The listing builds one solid part. Answer for the finished solid, in the listing's coordinates (mm). A direction names the side the tool comes from. Give positions to 0.01 mm unless a question says otherwise; leave off trailing zeros. Loops run counter-clockwise (first coordinate to the right, second up) from the corner with the lowest first, then second, coordinate; pieces in that order, holes last. Notation, with made-up numbers: M 44.5,1.5 L 82.5,1.5 A22 ccw 82.5,38.5 Z; hole C 75,41 d4. An arc over 180 degrees is marked long. Return JSON: item names as keys, results as strings.
from build123d import *

# Parameters (mm, degrees)
SKETCH_1_W          = 270
SKETCH_1_H          = 60
EXTRUDE_1_DEPTH     = 3
SKETCH_2_R          = 2.15
SKETCH_2_R_2        = 1.6
CUT_EXTRUDE_1_DEPTH = 3
SKETCH_3_R          = 1.6
CUT_EXTRUDE_2_DEPTH = 10
CUT_EXTRUDE_3_DEPTH = 10
FILLET_1_R          = 3
FILLET_2_R          = 4
SKETCH_5_W          = 100
SKETCH_5_H          = 40
CUT_EXTRUDE_4_DEPTH = 10
EXTRUDE_2_DEPTH     = 3
EXTRUDE_9_DEPTH     = 3
EXTRUDE_10_DEPTH    = 3
EXTRUDE_11_DEPTH    = 3
EXTRUDE_13_DEPTH    = 3
EXTRUDE_14_DEPTH    = 3
EXTRUDE_16_DEPTH    = 3
EXTRUDE_17_DEPTH    = 3
EXTRUDE_18_DEPTH    = 3
EXTRUDE_19_DEPTH    = 3
CUT_EXTRUDE_5_DEPTH = 4
FILLET_4_R          = 4


with BuildPart() as part:
    # 草图1 → 凸台-拉伸1 (new body)
    with BuildSketch(Plane(origin=(0, 0, 0), x_dir=(1, 0, 0), z_dir=(0, 1, 0))):
        Rectangle(SKETCH_1_W, SKETCH_1_H)
    extrude(amount=EXTRUDE_1_DEPTH)

    # 草图2 → 切除-拉伸1 (cut)
    with BuildSketch(Plane(origin=(0, 3, 0), x_dir=(1, 0, 0), z_dir=(0, 1, 0))):
        with Locations((-23, 0)):
            Circle(SKETCH_2_R)
        with Locations((23, 0)):
            Circle(SKETCH_2_R)
        with Locations((-125, -20)):
            Circle(SKETCH_2_R_2)
        with Locations((-125, -60)):
            Circle(SKETCH_2_R_2)
        with Locations((125, -60)):
            Circle(SKETCH_2_R_2)
        with Locations((125, -20)):
            Circle(SKETCH_2_R_2)
    extrude(amount=-CUT_EXTRUDE_1_DEPTH, mode=Mode.SUBTRACT)

    # 草图3 → 切除-拉伸2 (cut)
    with BuildSketch(Plane(origin=(0, 3, 0), x_dir=(1, 0, 0), z_dir=(0, 1, 0))):
        with Locations((125, 20)):
            Circle(SKETCH_3_R)
        with Locations((100, 20)):
            Circle(SKETCH_3_R)
        with Locations((75, 20)):
            Circle(SKETCH_3_R)
        with Locations((0, 20)):
            Circle(SKETCH_3_R)
        with Locations((-75, 20)):
            Circle(SKETCH_3_R)
        with Locations((-100, 20)):
            Circle(SKETCH_3_R)
        with Locations((-125, 20)):
            Circle(SKETCH_3_R)
    extrude(amount=-CUT_EXTRUDE_2_DEPTH, mode=Mode.SUBTRACT)

    # 草图4 → 切除-拉伸3 (cut)
    with BuildSketch(Plane(origin=(0, 3, 0), x_dir=(1, 0, 0), z_dir=(0, 1, 0))):
        with BuildLine():
            Line((-112.832473586, 10.419213325), (-112.99590583, 10.347711719))
            ThreePointArc((-112.99590583, 10.347711719), (-119.580786675, 12.924404223), (-117.00409417, 19.509285068))
            Line((-117.00409417, 19.509285068), (-116.840661926, 19.580786675))
            ThreePointArc((-116.840661926, 19.580786675), (-110.255781081, 17.00409417), (-112.832473586, 10.419213325))
        make_face()
        with BuildLine():
            Line((-79.771332565, 7.419213325), (-112.99590583, -7.116537478))
            ThreePointArc((-112.99590583, -7.116537478), (-119.580786675, -4.539844974), (-117.00409417, 2.045035871))
            Line((-117.00409417, 2.045035871), (-83.779520905, 16.580786675))
            ThreePointArc((-83.779520905, 16.580786675), (-77.194640061, 14.00409417), (-79.771332565, 7.419213325))
        make_face()
        with BuildLine():
            Line((-32.99590583, 10.419213325), (-112.99590583, -24.580786675))
            ThreePointArc((-112.99590583, -24.580786675), (-119.580786675, -22.00409417), (-117.00409417, -15.419213325))
            Line((-117.00409417, -15.419213325), (-37.00409417, 19.580786675))
            ThreePointArc((-37.00409417, 19.580786675), (-30.419213325, 17.00409417), (-32.99590583, 10.419213325))
        make_face()
        with BuildLine():
            Line((-32.99590583, -10.045035871), (-66.220479095, -24.580786675))
            ThreePointArc((-66.220479095, -24.580786675), (-72.805359939, -22.00409417), (-70.228667435, -15.419213325))
            Line((-70.228667435, -15.419213325), (-37.00409417, -0.883462522))
            ThreePointArc((-37.00409417, -0.883462522), (-30.419213325, -3.460155026), (-32.99590583, -10.045035871))
        make_face()
        with BuildLine():
            Line((-32.99590583, -24.509285068), (-33.159338074, -24.580786675))
            ThreePointArc((-33.159338074, -24.580786675), (-39.744218919, -22.00409417), (-37.167526414, -15.419213325))
            Line((-37.167526414, -15.419213325), (-37.00409417, -15.347711719))
            ThreePointArc((-37.00409417, -15.347711719), (-30.419213325, -17.924404223), (-32.99590583, -24.509285068))
        make_face()
        with BuildLine():
            Line((32.99590583, -24.509285068), (33.159338074, -24.580786675))
            ThreePointArc((33.159338074, -24.580786675), (39.744218919, -22.00409417), (37.167526414, -15.419213325))
            Line((37.167526414, -15.419213325), (37.00409417, -15.347711719))
            ThreePointArc((37.00409417, -15.347711719), (30.419213325, -17.924404223), (32.99590583, -24.509285068))
        make_face()
        with BuildLine():
            Line((32.99590583, -10.045035871), (66.220479095, -24.580786675))
            ThreePointArc((66.220479095, -24.580786675), (72.805359939, -22.00409417), (70.228667435, -15.419213325))
            Line((70.228667435, -15.419213325), (37.00409417, -0.883462522))
            ThreePointArc((37.00409417, -0.883462522), (30.419213325, -3.460155026), (32.99590583, -10.045035871))
        make_face()
        with BuildLine():
            Line((32.99590583, 10.419213325), (112.99590583, -24.580786675))
            ThreePointArc((112.99590583, -24.580786675), (119.580786675, -22.00409417), (117.00409417, -15.419213325))
            Line((117.00409417, -15.419213325), (37.00409417, 19.580786675))
            ThreePointArc((37.00409417, 19.580786675), (30.419213325, 17.00409417), (32.99590583, 10.419213325))
        make_face()
        with BuildLine():
            Line((79.771332565, 7.419213325), (112.99590583, -7.116537478))
            ThreePointArc((112.99590583, -7.116537478), (119.580786675, -4.539844974), (117.00409417, 2.045035871))
            Line((117.00409417, 2.045035871), (83.779520905, 16.580786675))
            ThreePointArc((83.779520905, 16.580786675), (77.194640061, 14.00409417), (79.771332565, 7.419213325))
        make_face()
        with BuildLine():
            Line((112.832473586, 10.419213325), (112.99590583, 10.347711719))
            ThreePointArc((112.99590583, 10.347711719), (119.580786675, 12.924404223), (117.00409417, 19.509285068))
            Line((117.00409417, 19.509285068), (116.840661926, 19.580786675))
            ThreePointArc((116.840661926, 19.580786675), (110.255781081, 17.00409417), (112.832473586, 10.419213325))
        make_face()
        Polygon((0, -20), (-22.5, -20), (0, 0), (22.5, -20), align=None)
    extrude(amount=-CUT_EXTRUDE_3_DEPTH, mode=Mode.SUBTRACT)

    # 圆角1
    fillet_1_edges = [part.edges().sort_by_distance(p)[0] for p in [
        (22.5, 1.5, 20),
        (-22.5, 1.5, 20),
        (0, 1.5, 0),
    ]]
    fillet(fillet_1_edges, radius=FILLET_1_R)

    # 圆角2
    fillet_2_edges = [part.edges().sort_by_distance(p)[0] for p in [
        (135, 1.5, 30),
        (-135, 1.5, 30),
        (-135, 1.5, -30),
        (135, 1.5, -30),
    ]]
    fillet(fillet_2_edges, radius=FILLET_2_R)

    # 草图5 → 切除-拉伸4 (cut)
    with BuildSketch(Plane(origin=(0, 3, 0), x_dir=(1, 0, 0), z_dir=(0, 1, 0))):
        with Locations((-85, -10)):
            Rectangle(SKETCH_5_W, SKETCH_5_H)
        with Locations((85, -10)):
            Rectangle(SKETCH_5_W, SKETCH_5_H)
    extrude(amount=-CUT_EXTRUDE_4_DEPTH, mode=Mode.SUBTRACT)

    # 草图6 → 凸台-拉伸2 (add)
    with BuildSketch(Plane(origin=(0, 3, 0), x_dir=(1, 0, 0), z_dir=(0, 1, 0))):
        with BuildLine():
            Line((-111.519942965, 10), (-118.153192546, 10))
            ThreePointArc((-118.153192546, 10), (-114.836567756, 21), (-111.519942965, 10))
        make_face()
    extrude(amount=-EXTRUDE_2_DEPTH)

    # 草图7 → 凸台-拉伸9 (add)
    with BuildSketch(Plane(origin=(0, 3, 0), x_dir=(1, 0, 0), z_dir=(0, 1, 0))):
        with BuildLine():
            Line((-98.821319018, 10), (-83.779520905, 16.580786675))
            ThreePointArc((-83.779520905, 16.580786675), (-78.241472851, 15.537113222), (-77.19285104, 10))
            Line((-77.19285104, 10), (-98.821319018, 10))
        make_face()
    extrude(amount=-EXTRUDE_9_DEPTH)

    # 草图8 → 凸台-拉伸10 (add)
    with BuildSketch(Plane(origin=(0, 3, 0), x_dir=(1, 0, 0), z_dir=(0, 1, 0))):
        with BuildLine():
            Line((-58.90303514, 10), (-35, 9.542422126))
            Line((-35, 9.542422126), (-32.99590583, 10.419213325))
            ThreePointArc((-32.99590583, 10.419213325), (-30.419213325, 17.00409417), (-37.00409417, 19.580786675))
            Line((-37.00409417, 19.580786675), (-58.90303514, 10))
        make_face()
    extrude(amount=-EXTRUDE_10_DEPTH)

    # 草图9 → 凸台-拉伸11 (add)
    with BuildSketch(Plane(origin=(0, 3, 0), x_dir=(1, 0, 0), z_dir=(0, 1, 0))):
        with BuildLine():
            Line((-35, -0.464249197), (-35, -10.921827071))
            Line((-35, -10.921827071), (-32.99590583, -10.045035871))
            ThreePointArc((-32.99590583, -10.045035871), (-30.105925349, -4.440514214), (-35, -0.464249197))
        make_face()
    extrude(amount=-EXTRUDE_11_DEPTH)

    # 草图10 → 凸台-拉伸13 (add)
    with BuildSketch(Plane(origin=(0, 3, 0), x_dir=(1, 0, 0), z_dir=(0, 1, 0))):
        with BuildLine():
            Line((-35, -14.928498393), (-35, -24.997328276))
            ThreePointArc((-35, -24.997328276), (-29.965585058, -19.962913335), (-35, -14.928498393))
        make_face()
    extrude(amount=-EXTRUDE_13_DEPTH)

    # 草图11 → 凸台-拉伸14 (add)
    with BuildSketch(Plane(origin=(0, 3, 0), x_dir=(1, 0, 0), z_dir=(0, 1, 0))):
        with BuildLine():
            Line((35, -0.464249197), (35, -10.921827071))
            ThreePointArc((35, -10.921827071), (29.771211063, -5.693038134), (35, -0.464249197))
        make_face()
    extrude(amount=-EXTRUDE_14_DEPTH)

    # 草图12 → 凸台-拉伸16 (add)
    with BuildSketch(Plane(origin=(0, 3, 0), x_dir=(1, 0, 0), z_dir=(0, 1, 0))):
        with BuildLine():
            Line((35, -14.928498393), (35, -24.997328276))
            ThreePointArc((35, -24.997328276), (29.965585058, -19.962913335), (35, -14.928498393))
        make_face()
    extrude(amount=-EXTRUDE_16_DEPTH)

    # 草图13 → 凸台-拉伸17 (add)
    with BuildSketch(Plane(origin=(0, 3, 0), x_dir=(1, 0, 0), z_dir=(0, 1, 0))):
        with BuildLine():
            Line((58.90303514, 10), (37.00409417, 19.580786675))
            ThreePointArc((37.00409417, 19.580786675), (30.419213325, 17.00409417), (32.99590583, 10.419213325))
            Line((32.99590583, 10.419213325), (35, 9.542422126))
            Line((35, 9.542422126), (58.90303514, 10))
        make_face()
    extrude(amount=-EXTRUDE_17_DEPTH)

    # 草图14 → 凸台-拉伸18 (add)
    with BuildSketch(Plane(origin=(0, 3, 0), x_dir=(1, 0, 0), z_dir=(0, 1, 0))):
        with BuildLine():
            Line((98.821319018, 10), (83.779520905, 16.580786675))
            ThreePointArc((83.779520905, 16.580786675), (78.241472851, 15.537113222), (77.19285104, 10))
            Line((77.19285104, 10), (98.821319018, 10))
        make_face()
    extrude(amount=-EXTRUDE_18_DEPTH)

    # 草图15 → 凸台-拉伸19 (add)
    with BuildSketch(Plane(origin=(0, 3, 0), x_dir=(1, 0, 0), z_dir=(0, 1, 0))):
        with BuildLine():
            Line((116.732439942, 10), (112.940695569, 10))
            ThreePointArc((112.940695569, 10), (114.836567756, 20.347366768), (116.732439942, 10))
        make_face()
    extrude(amount=-EXTRUDE_19_DEPTH)

    # 草图16 → 切除-拉伸5 (cut, through all)
    with BuildSketch(Plane(origin=(0, 3, 0), x_dir=(1, 0, 0), z_dir=(0, 1, 0))):
        with BuildLine():
            Line((-23.5, 17), (-51.5, 17))
            ThreePointArc((-51.5, 17), (-54.5, 20), (-51.5, 23))
            Line((-51.5, 23), (-23.5, 23))
            ThreePointArc((-23.5, 23), (-20.5, 20), (-23.5, 17))
        make_face()
        with BuildLine():
            Line((23.5, 17), (51.5, 17))
            ThreePointArc((51.5, 17), (54.5, 20), (51.5, 23))
            Line((51.5, 23), (23.5, 23))
            ThreePointArc((23.5, 23), (20.5, 20), (23.5, 17))
        make_face()
    extrude(amount=-CUT_EXTRUDE_5_DEPTH, mode=Mode.SUBTRACT)

    # 圆角4
    fillet_4_edges = [part.edges().sort_by_distance(p)[0] for p in [
        (35, 1.5, -9.542422126),
        (-135, 1.5, -10),
        (-35, 1.5, -9.542422126),
        (-35, 1.5, 30),
        (35, 1.5, 30),
        (135, 1.5, -10),
    ]]
    fillet(fillet_4_edges, radius=FILLET_4_R)


solid = part.part
(1) The part is cut by section B-B (y = 1.5). Give the number of separate pieces and of enclosed holes in the cut face, and give its area (3 significant figures).
Values follow:
{"separate pieces": "1", "enclosed holes": "12", "area": "7,300 mm²"}
(2) Determine the mould class of faces 3 (the flat face through (-2, 0, -7)), 4 (the cylindrical face through (25.05, 1.52, -0.65)), 5 (the flat face through (9, 2, 8)) for opening direction X: released by +X, released by -X, zero draft, split by the parting line, or undercut.
Values follow:
{"face 3": "zero draft", "face 4": "undercut", "face 5": "undercut"}
(3) The part is cut by section A-A (z = 6). Determine the outline of the cut face in (x, y).
Values follow:
{"outline": "M -35,0 L -6.75,0 L -6.75,3 L -35,3 Z; M 6.75,0 L 35,0 L 35,3 L 6.75,3 Z"}
(4) A tool of negligible diameter and unlimited length cuts with its end or side. For faces 1 (the flat face through (-9, 2, 8)), 2 (the flat face through (-2, 3, -7)), from which of +Z, -Z, +X, -X, +Y, -Y can it reach the whole face along a straight path? Write none if from no direction.
Values follow:
{"face 1": "+Y, -Y", "face 2": "+Z, -Z, +X, -X, +Y"}
(5) Straight lines are drawn through the part: line 1 along Z through (x, y) = (0, 1.5); line 2 along Z through (x, y) = (-125, 2.4); line 3 along X through (y, z) = (2.2, 0). For each, find the intervals that lie inside material, in ascending order.
Values follow:
{"line 1": "-30 to -21.6, -18.4 to 1.01, 20 to 30", "line 2": "-30 to -21.6, -18.4 to -10", "line 3": "-35 to -25.15, -20.85 to 20.85, 25.15 to 35"}
(6) Given pin 1 (3 mm diameter, centred on x = 125, z = -20, fed in from -Y); pin 2 (1.5 mm diameter, centred on y = 1, z = 3.5, fed in from -X); pin 3 (1.5 mm diameter, centred on x = -111.5, y = 2, fed in from +Z); pin 4 (0.9 mm diameter, centred on x = -36, y = 1, fed in from +Z), each flat-ended and moving along its own axis, determine where each tip first touches the part or whether it passes through.
Values follow:
{"pin 1": "through", "pin 2": "x = -35", "pin 3": "z = -10", "pin 4": "z = -7.64"}
(7) The part is cut by section C-C (x = -69). Determine the outline of the cut face in (y, z), and give its area (3 significant figures).
Values follow:
{"outline": "M 0,-30 L 3,-30 L 3,-10 L 0,-10 Z", "area": "60.0 mm²"}
